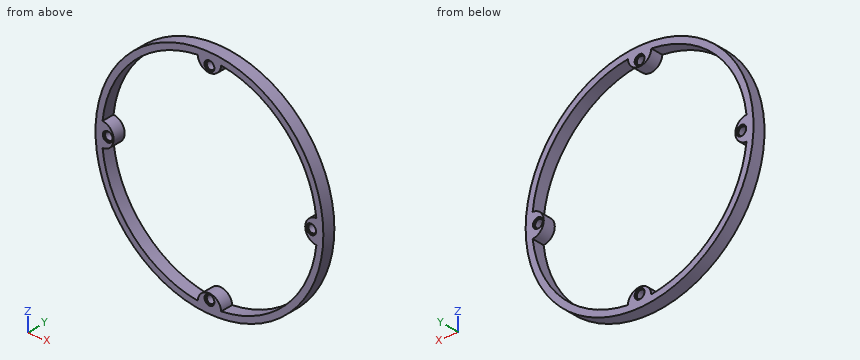
from build123d import *

# Parameters (mm, degrees)
F0_R     = 71.5
F0_R_2   = 2.4
F1_DEPTH = 3.88
F2_R     = 3.1
F3_DEPTH = 0.8
F4_R     = 3.1
F5_DEPTH = 0.8


with BuildPart() as f1:
    # F0 (on Front) → F1 (new body, symmetric)
    with BuildSketch(Plane.XZ):
        Circle(F0_R)
        with Locations((0, -63.81)):
            Circle(F0_R_2, mode=Mode.SUBTRACT)
        with Locations((-63.81, 0)):
            Circle(F0_R_2, mode=Mode.SUBTRACT)
        with BuildLine():
            ThreePointArc((-67.09656, 7.368964), (-47.729708, 47.729708), (-7.368964, 67.09656))
            ThreePointArc((-7.368964, 67.09656), (0, 60.12), (7.368964, 67.09656))
            ThreePointArc((7.368964, 67.09656), (47.729708, 47.729708), (67.09656, 7.368964))
            ThreePointArc((67.09656, 7.368964), (60.12, 0), (67.09656, -7.368964))
            ThreePointArc((67.09656, -7.368964), (47.729708, -47.729708), (7.368964, -67.09656))
            ThreePointArc((7.368964, -67.09656), (0, -60.12), (-7.368964, -67.09656))
            ThreePointArc((-7.368964, -67.09656), (-47.729708, -47.729708), (-67.09656, -7.368964))
            ThreePointArc((-67.09656, -7.368964), (-60.12, 0), (-67.09656, 7.368964))
        make_face(mode=Mode.SUBTRACT)
        with Locations((63.81, 0)):
            Circle(F0_R_2, mode=Mode.SUBTRACT)
        with Locations((0, 63.81)):
            Circle(F0_R_2, mode=Mode.SUBTRACT)
    extrude(amount=F1_DEPTH, both=True)

    # F2 (on face) → F3 (cut)
    with BuildSketch(Plane.XZ.offset(3.88)):
        with Locations((0, 63.81)):
            Circle(F2_R)
        with Locations((63.81, 0)):
            Circle(F2_R)
        with Locations((0, -63.81)):
            Circle(F2_R)
        with Locations((-63.81, 0)):
            Circle(F2_R)
    extrude(amount=-F3_DEPTH, mode=Mode.SUBTRACT)

    # F4 (on face) → F5 (cut)
    with BuildSketch(Plane(origin=(0, 3.88, 0), x_dir=(-1, 0, 0), z_dir=(0, 1, 0))):
        with Locations((0, 63.81)):
            Circle(F4_R)
        with Locations((63.81, 0)):
            Circle(F4_R)
        with Locations((0, -63.81)):
            Circle(F4_R)
        with Locations((-63.81, 0)):
            Circle(F4_R)
    extrude(amount=-F5_DEPTH, mode=Mode.SUBTRACT)


solid = f1.part
Work out the finished part from the listing and answer in its coordinate system (mm). Give positions to 0.01 mm unless a question says otherwise; leave off trailing zeros. Write each loop counter-clockwise with the first axis right and the second up, starting at its lowest first coordinate (ties: lowest second). Pieces come first, ordered by that corner, then holes. Notation, with made-up numbers: (26, -24.5) - (54, -24.5) arc R21 cw to (54, 14.5) - close; hole circle Ø5 at (-33.75, 52.25). An arc over 180 degrees is marked (long way). One line per item, written item: value. Start each with the question number.
1. Find section C-C (y = -1.5). Write down the section's boundary in (x, z).
2. Find section D-D (x = -23). Write down the section's boundary in (y, z).
3. Find section A-A (x = 0). State how many separate pieces and enclosed holes the cut face has, then the cut area to 3 significant figures.
4. Consider probe 1 along Z at (x, y) = (-35.5, 1.25); probe 2 along X at (y, z) = (3.5, 29.5); probe 3 along Z at (x, y) = (8, -2.75). Determine where each line is inside the solid, lowest interval first.
5. Given pin 1 (6 mm diameter, centred on x = -63.81, z = 0, fed in from +Y); pin 2 (3 mm diameter, centred on x = -62.5, z = 0, fed in from -Y); pin 3 (1 mm diameter, centred on y = -3, z = -14, fed in from -X); pin 4 (7 mm diameter, centred on x = -1, z = 63, fed in from +Y), each flat-ended and moving along its own axis, determine where each tip first touches the part or whether it passes through.
Geometry results:
1. outline: circle Ø143 at (0, 0); hole (-67.1, -7.37) arc R67.5 ccw to (-7.37, -67.1) arc R7.38 cw to (7.37, -67.1) arc R67.5 ccw to (67.1, -7.37) arc R7.38 cw to (67.1, 7.37) arc R67.5 ccw to (7.37, 67.1) arc R7.38 cw to (-7.37, 67.1) arc R67.5 ccw to (-67.1, 7.37) arc R7.38 cw to start; hole circle Ø4.8 at (-63.81, 0); hole circle Ø4.8 at (0, -63.81); hole circle Ø4.8 at (0, 63.81); hole circle Ø4.8 at (63.81, 0)
2. outline: (-3.88, -67.7) - (3.88, -67.7) - (3.88, -63.46) - (-3.88, -63.46) - close; (-3.88, 63.46) - (3.88, 63.46) - (3.88, 67.7) - (-3.88, 67.7) - close
3. separate pieces: 4
3. enclosed holes: 0
3. area: 97.6 mm2
4. probe 1: -62.06 to -57.41, 57.41 to 62.06
4. probe 2: -65.13 to -60.71, 60.71 to 65.13
4. probe 3: -71.05 to -67.02, 67.02 to 71.05
5. pin 1: y = 3.08
5. pin 2: y = -3.08
5. pin 3: x = -70.21
5. pin 4: y = 3.88
